Source: CAD feature listing. Evaluate the final solid. Frame: model axes, mm. Give positions to 0.01 mm unless a question says otherwise; leave off trailing zeros. Write each loop counter-clockwise with the first axis right and the second up, starting at its lowest first coordinate (ties: lowest second). Pieces come first, ordered by that corner, then holes. Notation, with made-up numbers: (2, 79) -> (42, 79) arc R15 cw to (42, 98) -> close; hole circle Ø7 at (81.5, 44.5). An arc over 180 degrees is marked (long way). Answer as a JSON object with one key per item and string values. Group by question number.
Item 1: First-contact query: pin 1 Ø1.8 at (y, z) = (0.5, 2.5) entering from -X; pin 2 Ø2 at (x, y) = (36, 0.5) entering from +Z; pin 3 Ø1.8 at (y, z) = (0, 4) entering from +X. Flat tips, straight axial feed; report the tip coordinate or a pass-through.
Item 2: Section query A-A on x = 12. Return the cut outline in (y, z), plus the area to 3 significant figures.
Item 3: Ray query, probe 1 along X at (y, z) = (-0.3, 3.5); probe 2 along Y at (x, z) = (-9.5, 0.25); probe 3 along X at (y, z) = (0.6, 2.2). Return the intervals inside material, ascending. Write a range as from..to.
from build123d import *

# Parameters (mm, degrees)
SKICA2_W                 = 150
SKICA2_H                 = 4.2
SKICA2_W_2               = 18
SKICA2_H_2               = 1
P_IDAT_VYSUNUT_M2_DEPTH  = 0.8
SKICA3_R                 = 1.5
SKICA3_R_2               = 1.75
P_IDAT_VYSUNUT_M3_DEPTH  = 2.2
SKICA5_R                 = 1.9
P_IDAT_VYSUNUT_M5_DEPTH  = 2
ZKOSEN_2_SIZE            = 1.5
SKICA7_W                 = 1
SKICA7_H                 = 5
ODEBRAT_VYSUNUT_M1_DEPTH = 4


with BuildPart() as part:
    # Skica2 → Přidat vysunutím2 (new body)
    with BuildSketch(Plane.XY):
        Rectangle(SKICA2_W, SKICA2_H)
        with Locations((-5, -0.2)):
            Rectangle(SKICA2_W_2, SKICA2_H_2, mode=Mode.SUBTRACT)
    extrude(amount=P_IDAT_VYSUNUT_M2_DEPTH)

    # Skica3 → Přidat vysunutím3 (add)
    with BuildSketch(Plane.XY.offset(0.8)):
        with Locations((-50, -0.2)):
            Circle(SKICA3_R)
        with Locations((50, 0)):
            Circle(SKICA3_R_2)
    extrude(amount=P_IDAT_VYSUNUT_M3_DEPTH)

    # Skica5 → Přidat vysunutím5 (add)
    with BuildSketch(Plane.XY.offset(3)):
        with Locations((-50, -0.2)):
            Circle(SKICA5_R)
        with Locations((50, 0)):
            Circle(SKICA5_R)
    extrude(amount=P_IDAT_VYSUNUT_M5_DEPTH)

    # Zkosení2
    zkosen_2_edges = [part.edges().sort_by_distance(p)[0] for p in [
        (-51.9, -0.2, 5),
        (48.1, 0, 5),
    ]]
    chamfer(zkosen_2_edges, length=ZKOSEN_2_SIZE)

    # Skica7 → Odebrat vysunutím1 (cut)
    with BuildSketch(Plane.XY.offset(5)):
        with Locations((-50, -0.2)):
            Rectangle(SKICA7_W, SKICA7_H)
        with Locations((50, 0)):
            Rectangle(SKICA7_W, SKICA7_H)
    extrude(amount=-ODEBRAT_VYSUNUT_M1_DEPTH, mode=Mode.SUBTRACT)


solid = part.part
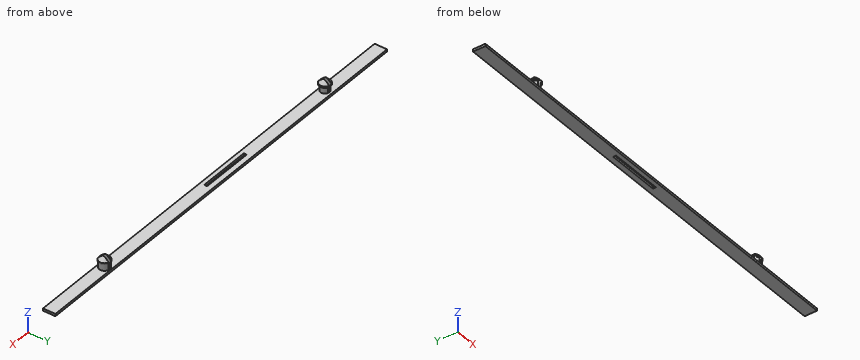
Worked answers:
{
 "1": {"pin 1": "x = -51.9", "pin 2": "z = 0.8", "pin 3": "x = 51.9"},
 "2": {"outline": "(-2.1, 0) -> (2.1, 0) -> (2.1, 0.8) -> (-2.1, 0.8) -> close", "area": "3.36 mm^2"},
 "3": {"probe 1": "-51.9..-50.5, -49.5..-48.1, 48.12..49.5, 50.5..51.88", "probe 2": "-2.1..-0.7, 0.3..2.1", "probe 3": "-51.27..-50.5, -49.5..-48.73, 48.36..49.5, 50.5..51.64"}
}
